```python
from build123d import *

# Parameters (mm, degrees)
SKETCH2_W                     = 31.75
SKETCH2_H                     = 29.845
BOSS_EXTRUDE1_DEPTH           = 3.175
F_0_16_4_064_DIAMETER_HOLE1_D = 4.064


with BuildPart() as part:
    # Sketch2 → Boss-Extrude1 (new body)
    with BuildSketch(Plane.XY):
        with Locations((15.875, 14.9225)):
            Rectangle(SKETCH2_W, SKETCH2_H)
        with BuildLine():
            Line((2.775, 9.8425), (2.775, 20.0025))
            ThreePointArc((2.775, 20.0025), (3.875, 21.1025), (4.975, 20.0025))
            Line((4.975, 20.0025), (4.975, 9.8425))
            ThreePointArc((4.975, 9.8425), (3.875, 8.7425), (2.775, 9.8425))
        make_face(mode=Mode.SUBTRACT)
        with BuildLine():
            Line((28.975, 9.8425), (28.975, 20.0025))
            ThreePointArc((28.975, 20.0025), (27.875, 21.1025), (26.775, 20.0025))
            Line((26.775, 20.0025), (26.775, 9.8425))
            ThreePointArc((26.775, 9.8425), (27.875, 8.7425), (28.975, 9.8425))
        make_face(mode=Mode.SUBTRACT)
    extrude(amount=BOSS_EXTRUDE1_DEPTH)

    # Ø0.16 (4.064) Diameter Hole1 (through all)
    with Locations(Plane(origin=(0, 0, 0), x_dir=(-1, 0, 0), z_dir=(0, 0, -1))):
        with Locations((-25.4, 24.4475), (-6.35, 24.4475), (-6.35, 5.3975), (-25.4, 5.3975)):
            Hole(F_0_16_4_064_DIAMETER_HOLE1_D / 2)


solid = part.part
```
The model under review builds one solid part; all positions refer to its coordinate system, in mm. A direction names the side the tool comes from. Coordinates: 2 decimals unless noted, no trailing zeros. Write each loop counter-clockwise with the first axis right and the second up, starting at its lowest first coordinate (ties: lowest second). Pieces come first, ordered by that corner, then holes.
1) We need section A-A on y = 19.5. State the section outline as (x, z) points (3 decimals), then the cut area to 3 significant figures.
2) To check wall thickness, follow probe 1 along Y at (x, z) = (6.5, 2.2) (3 decimals); probe 2 along X at (y, z) = (16.5, 0.9) (3 decimals); probe 3 along X at (y, z) = (23, 0.65). State the ranges of each line that lie inside material, in increasing order.
3) Machinability: for faces 1 (the face through (2.775, 15, 2)), 2 (the face through (16, 15, 3.175)), which of the approach directions +Z, -Z, +X, -X, +Y, -Y give a long, thin tool a straight path to every point of the face, cutting with its end or side? Answer none if there is none.
4) We need section B-B on x = 6.35. State the section outline as (y, z) points (1 decimal), then the cut area to 3 significant figures.
5) We need section C-C on z = 0.6. Count the separate pieces of the cut face and the enclosed holes in it, then the cut area to 3 significant figures.
6) Clearance check with a flat-ended pin moving along its axis: pin 1 Ø5.5 at (x, y) = (6.35, 24.45) entering from -Z. State where the tip first meets the part, or that it passes through.
7) The part is to be moulded in two halves that separate along Y. For faces 3 (the face through (16, 0, 2)), 4 (the face through (27.851, 8.743, 1.565)), 5 (the face through (0, 15, 2)), say which applies: pulls with the +Y half, pulls with the -Y half, needs draft (parallel to the pull), parting line crosses it, or undercut.
Answer list:
1. outline: (0, 0) - (2.775, 0) - (2.775, 3.175) - (0, 3.175) - close; (4.975, 0) - (26.775, 0) - (26.775, 3.175) - (4.975, 3.175) - close; (28.975, 0) - (31.75, 0) - (31.75, 3.175) - (28.975, 3.175) - close
1. area: 86.8 mm2
2. probe 1: y = 0 to 3.371, 7.424 to 22.421, 26.474 to 29.845
2. probe 2: x = 0 to 2.775, 4.975 to 26.775, 28.975 to 31.75
2. probe 3: x = 0 to 4.92, 7.78 to 23.97, 26.83 to 31.75
3. face 1: +Z, -Z
3. face 2: +Z, +X, -X, +Y, -Y
4. outline: (0, 0) - (3.4, 0) - (3.4, 3.2) - (0, 3.2) - close; (7.4, 0) - (22.4, 0) - (22.4, 3.2) - (7.4, 3.2) - close; (26.5, 0) - (29.8, 0) - (29.8, 3.2) - (26.5, 3.2) - close
4. area: 69.0 mm2
5. separate pieces: 1
5. enclosed holes: 6
5. area: 843 mm2
6. pin 1: stops at z = 0
7. face 3: pulls with the -Y half
7. face 4: undercut
7. face 5: needs draft
